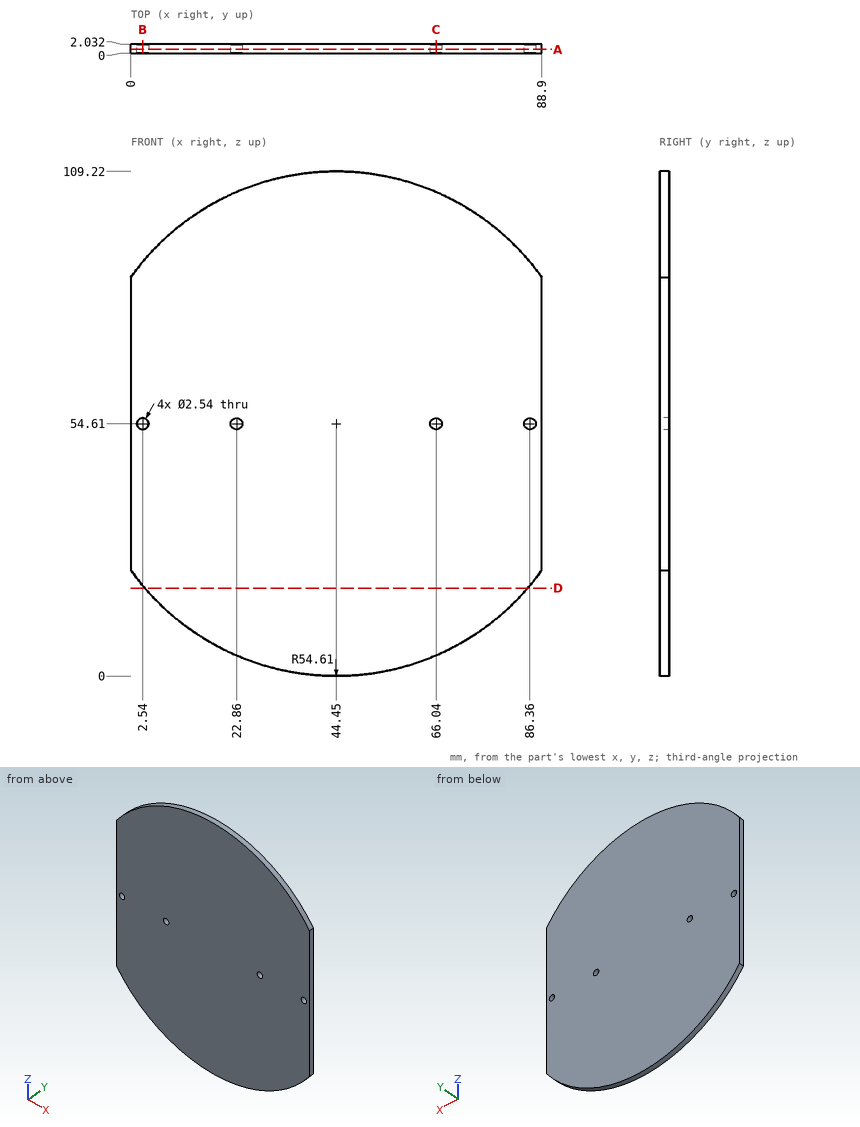
Print and shaded views of the part. All mm, measured from the part's lowest x, y and z. Coordinates: 2 decimals unless noted, no trailing zeros. Order: outer loops, then holes, each group sorted by start corner. A loop starts at its lowest first (then second) coordinate and runs counter-clockwise, first axis right, second up. Notation, with made-up numbers: (-12.5, 30) - (38.5, 30) arc R3 cw to (38.5, 34) - close; hole circle Ø4 at (-18.5, -40). An arc over 180 degrees is marked (long way). Return JSON: item names as keys, results as strings. Group by question number.
Item 1: Pin check, flat tip, straight feed: pin 1 (2 mm diameter, centred on x = 17, z = 73, fed in from -Y). Stop position of the tip, or through.
Item 2: Cut at A-A (y = 0.85). List the corners of the cut face in (x, z), plus the area to 3 significant figures.
Item 3: Cut at B-B (x = 2.54). List the corners of the cut face in (y, z).
Item 4: Cut at C-C (x = 66.04). List the corners of the cut face in (y, z).
Item 5: Drill centre lines: probe 1 along Z at (x, y) = (22.86, 0.6); probe 2 along Z at (x, y) = (86.36, 1.5); probe 3 along Z at (x, y) = (46, 0.6). Where is each one in solid material? Low to high. Write a range as from..to.
Item 6: Cut at D-D (z = 19). List the corners of the cut face in (x, y).
Check values:
{
 "1": {"pin 1": "stops at y = 0"},
 "2": {"outline": "(0, 22.89) arc R54.61 ccw to (88.9, 22.89) - (88.9, 86.33) arc R54.61 ccw to (0, 86.33) - close; hole circle Ø2.54 at (2.54, 54.61); hole circle Ø2.54 at (22.86, 54.61); hole circle Ø2.54 at (66.04, 54.61); hole circle Ø2.54 at (86.36, 54.61)", "area": "8,470 mm2"},
 "3": {"outline": "(0, 19.6) - (2.03, 19.6) - (2.03, 53.34) - (0, 53.34) - close; (0, 55.88) - (2.03, 55.88) - (2.03, 89.62) - (0, 89.62) - close"},
 "4": {"outline": "(0, 4.45) - (2.03, 4.45) - (2.03, 53.34) - (0, 53.34) - close; (0, 55.88) - (2.03, 55.88) - (2.03, 104.77) - (0, 104.77) - close"},
 "5": {"probe 1": "z = 4.45..53.34, 55.88..104.77", "probe 2": "z = 19.6..53.34, 55.88..89.62", "probe 3": "z = 0.02..109.2"},
 "6": {"outline": "(3.05, 0) - (85.85, 0) - (85.85, 2.03) - (3.05, 2.03) - close"}
}
